Read the model definition and answer for the solid it produces. Units are mm, in the model's axes. Round coordinates to 2 decimals unless told otherwise and drop trailing zeros. Write each loop counter-clockwise with the first axis right and the second up, starting at its lowest first coordinate (ties: lowest second). Pieces come first, ordered by that corner, then holes. Notation, with made-up numbers: (54, 62) -> (93, 62) arc R13 cw to (93, 70) -> close; hole circle Ø1 at (-20, 19). An arc over 180 degrees is marked (long way). Return JSON: item names as keys, results as strings. Group by question number.
(1) Given pin 1 (1.5 mm diameter, centred on y = -3, z = 2, fed in from +X), flat-ended and moving along its own axis, determine where the tip first touches the part or whether it passes through.
(2) A cutting plane is placed at D-D on x = -2.2. Give the vertices of the cut face in (y, z).
(3) A cutting plane is placed at C-C on y = -8.75. Give the vertices of the cut face in (x, z), then the cut area to 3 significant figures.
(4) A cutting plane is placed at A-A on x = 0. Give the vertices of the cut face in (y, z).
(5) The mould has two halves that part along Z. Classify faces 1 (the flat face through (1, -15, -1)), 2 (the cylindrical face through (-0.54, -7.4, -2.44)), 3 (the flat face through (0, -14.6, 0)): released by +Z, released by -Z, zero draft, split by the parting line, or undercut.
(6) A cutting plane is placed at B-B on z = 0. Give the vertices of the cut face in (x, y), then the cut area to 3 significant figures.
(7) Straight lines are drawn through the part: line 1 (Z direction, x = -0.1, y = -1.75); line 2 (X direction, y = -6, z = 2). For each, find the intervals that lie inside material, in ascending order.
```python
from build123d import *

# Parameters (mm, degrees)
F0_W     = 120
F0_H     = 4
F1_DEPTH = 4
F3_R     = 2.5
F4_DEPTH = 15
F5_W     = 0.4
F5_H     = 0.4
F5_H_2   = 1.1
F5_W_2   = 1.1
F6_DEPTH = 0.4


with BuildPart() as f1:
    # F0 (on Top) → F1 (new body)
    with BuildSketch(Plane.XY):
        Polygon((-79.6833248483, 0), (-93.6833248483, 0), (-93.6833248483, -12), (-79.6833248483, -12), (-79.6833248483, -8), (-79.6833248483, -4), align=None)
        with Locations((-19.6833248483, -2)):
            Rectangle(F0_W, F0_H)
        Polygon((54.3166751517, 0), (40.3166751517, 0), (40.3166751517, -4), (40.3166751517, -8), (40.3166751517, -12), (54.3166751517, -12), align=None)
        with Locations((-19.6833248483, -10)):
            Rectangle(F0_W, F0_H)
    extrude(amount=F1_DEPTH)


with BuildPart() as f4:
    # F3 (on Front) → F4 (new body)
    with BuildSketch(Plane.XZ):
        Circle(F3_R)
    extrude(amount=F4_DEPTH)

    # F5 (on face) → F6 (cut)
    with BuildSketch(Plane.XZ.offset(15)):
        with Locations((-0.2, 0.2)):
            Rectangle(F5_W, F5_H)
        with Locations((0.2, -0.2)):
            Rectangle(F5_W, F5_H)
        with Locations((-0.2, -0.2)):
            Rectangle(F5_W, F5_H)
        with Locations((0.2, 0.2)):
            Rectangle(F5_W, F5_H)
        with Locations((-0.2, 0.95)):
            Rectangle(F5_W, F5_H_2)
        with Locations((0.2, 0.95)):
            Rectangle(F5_W, F5_H_2)
        with Locations((0.2, -0.95)):
            Rectangle(F5_W, F5_H_2)
        with Locations((-0.2, -0.95)):
            Rectangle(F5_W, F5_H_2)
        with Locations((-0.95, -0.2)):
            Rectangle(F5_W_2, F5_H)
        with Locations((-0.95, 0.2)):
            Rectangle(F5_W_2, F5_H)
        with Locations((0.95, 0.2)):
            Rectangle(F5_W_2, F5_H)
        with Locations((0.95, -0.2)):
            Rectangle(F5_W_2, F5_H)
    extrude(amount=-F6_DEPTH, mode=Mode.SUBTRACT)


solid = f4.part
```
Checks:
{
 "1": {"pin 1": "stops at x = 2.17"},
 "2": {"outline": "(-15, -1.19) -> (0, -1.19) -> (0, 1.19) -> (-15, 1.19) -> close"},
 "3": {"outline": "circle Ø5 at (0, 0)", "area": "19.6 mm^2"},
 "4": {"outline": "(-15, -2.5) -> (0, -2.5) -> (0, 2.5) -> (-15, 2.5) -> (-15, 1.5) -> (-14.6, 1.5) -> (-14.6, -1.5) -> (-15, -1.5) -> close"},
 "5": {"face 1": "zero draft", "face 2": "split by the parting line", "face 3": "undercut"},
 "6": {"outline": "(-2.5, -15) -> (-1.5, -15) -> (-1.5, -14.6) -> (1.5, -14.6) -> (1.5, -15) -> (2.5, -15) -> (2.5, 0) -> (-2.5, 0) -> close", "area": "73.8 mm^2"},
 "7": {"line 1": "z = -2.5 to 2.5", "line 2": "x = -1.5 to 1.5"}
}
